```python
from build123d import *

# Parameters (mm, degrees)
FILLET_1_R = 0.4


with BuildPart() as part:
    # Эскиз1 → Повернуть1 (revolve)
    with BuildSketch(Plane(origin=(0, 0, 0), x_dir=(0, 0, -1), z_dir=(1, 0, 0))):
        Polygon((-2, 7), (-2, 9), (0, 9), (0, 4.5), (-31, 4.5), (-31, 3), (-35, 3), (-35, 7), align=None)
    revolve(axis=Axis((0, 0, -80.9), (0, 0, 1)))

    # Скругление1
    fillet_1_edges = [part.edges().sort_by_distance(p)[0] for p in [
        (0, -7, 35),
        (0, -9, 0),
    ]]
    fillet(fillet_1_edges, radius=FILLET_1_R)


solid = part.part
```
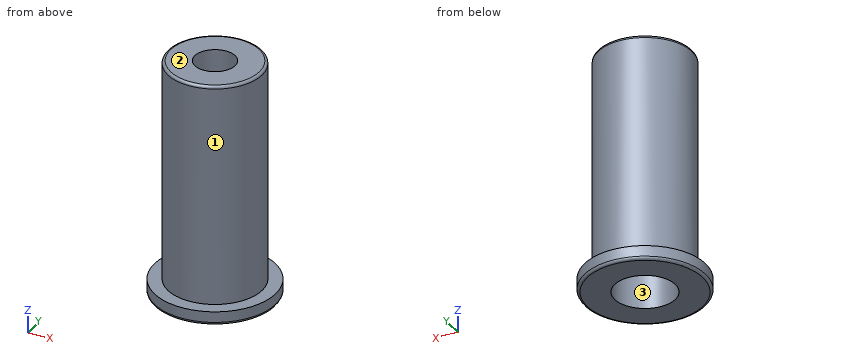
Check sheet for the modelled part. Datum: model origin and axes. Units: mm. Face numbers are marked on the shaded views. Give positions to 0.01 mm unless a question says otherwise; leave off trailing zeros. Write each loop counter-clockwise with the first axis right and the second up, starting at its lowest first coordinate (ties: lowest second). Pieces come first, ordered by that corner, then holes. Notation, with made-up numbers: (42, 88.5) - (60, 88.5) arc R21 cw to (60, 113.5) - close; hole circle Ø1 at (56.25, 15). An arc over 180 degrees is marked (long way). Answer as a JSON object with one key per item and string values. Group by question number.
1) Thickness scan on probe 1 along Y at (x, z) = (0.25, 4); probe 2 along X at (y, z) = (0, 17); probe 3 along X at (y, z) = (0, 31.9). Record the ranges inside material, lowest first. Write a range as from..to.
2) Depth check by flat-ended pin: P1, Ø6, axis at x = 2.5, z = 17, coming from the +Y side; P2, Ø6, axis at y = 0, z = 18.5, coming from the -X side; P3, Ø8, axis at x = -4, z = 23, coming from the -Y side. Enter the tip coordinate at first touch or a pass-through.
3) Release check for a two-part mould opening along X. For the marked faces 1, 2 and 3 record: pulls with the +X half, pulls with the -X half, needs draft (parallel to the pull), parting line crosses it, or undercut.
4) Sectioned sample at C-C (z = 16). Record the cut outline in (x, y), then the cut area to 3 significant figures.
5) Sectioned sample at A-A (y = 0). Record the cut outline in (x, z), then the cut area to 3 significant figures.
Geometry results:
{
 "1": {"probe 1": "y = -7..-4.49, 4.49..7", "probe 2": "x = -7..-4.5, 4.5..7", "probe 3": "x = -7..-3, 3..7"},
 "2": {"P1": "stops at y = 7", "P2": "stops at x = -7", "P3": "stops at y = -7"},
 "3": {"face 1": "parting line crosses it", "face 2": "needs draft", "face 3": "undercut"},
 "4": {"outline": "circle Ø14 at (0, 0); hole circle Ø9 at (0, 0)", "area": "90.3 mm^2"},
 "5": {"outline": "(-9, 0.4) arc R0.4 ccw to (-8.6, 0) - (-4.5, 0) - (-4.5, 31) - (-3, 31) - (-3, 35) - (-6.6, 35) arc R0.4 ccw to (-7, 34.6) - (-7, 2) - (-9, 2) - close; (3, 31) - (4.5, 31) - (4.5, 0) - (8.6, 0) arc R0.4 ccw to (9, 0.4) - (9, 2) - (7, 2) - (7, 34.6) arc R0.4 ccw to (6.6, 35) - (3, 35) - close", "area": "195 mm^2"}
}
